```python
from build123d import *

# Parameters (mm, degrees)
BOSS_EXTRUDE1_DEPTH = 6.35
CUT_EXTRUDE2_START  = -7.35
CUT_EXTRUDE2_DEPTH  = 8.35
CIRPATTERN2_COUNT   = 8
CIRPATTERN2_ANGLE   = 180


with BuildPart() as part:
    # Sketch1 → Boss-Extrude1 (new body)
    with BuildSketch(Plane(origin=(0, 0, 0), x_dir=(0, 0, -1), z_dir=(1, 0, 0))):
        with BuildLine():
            Line((-60.325, -98.425), (-60.325, 1.27))
            ThreePointArc((-60.325, 1.27), (-12.969041148, 54.83761073), (46.001592655, 14.408164693))
            Line((46.001592655, 14.408164693), (54.245104063, -18.439722464))
            ThreePointArc((54.245104063, -18.439722464), (49.680727349, -26.131903505), (41.952464165, -21.628889834))
            Line((41.952464165, -21.628889834), (33.734959483, 9.03925515))
            ThreePointArc((33.734959483, 9.03925515), (-4.558627263, 34.626211783), (-34.925, 0))
            Line((-34.925, 0), (-34.925, -98.425))
            ThreePointArc((-34.925, -98.425), (-47.625, -111.125), (-60.325, -98.425))
        make_face()
    extrude(amount=BOSS_EXTRUDE1_DEPTH)

    # Sketch5 → Cut-Extrude2 (cut)
    with BuildSketch(Plane(origin=(6.35, 0, 0), x_dir=(0, 0, -1), z_dir=(1, 0, 0)).offset(CUT_EXTRUDE2_START)):
        Polygon((-38.1, 6.35), (-41.275, 6.35), (-41.275, 0), (-35.06174314, 0), (-35.06174314, 6.35), align=None)
    cut_extrude2 = extrude(amount=CUT_EXTRUDE2_DEPTH, mode=Mode.SUBTRACT)

    # CirPattern2: Cut-Extrude2 ×8 about axis, 4 skipped
    cirpattern2_axis = Axis((0, 0, 0), (-1, 0, 0))
    add([cut_extrude2.rotate(cirpattern2_axis, i * CIRPATTERN2_ANGLE / (CIRPATTERN2_COUNT - 1)) for i in range(1, CIRPATTERN2_COUNT) if i not in (2, 3, 4, 7)], mode=Mode.SUBTRACT)


solid = part.part
```
The listing builds one solid part. Answer for the finished solid, in the listing's coordinates (mm). A direction names the side the tool comes from. Round coordinates to 2 decimals unless told otherwise and drop trailing zeros. Write each loop counter-clockwise with the first axis right and the second up, starting at its lowest first coordinate (ties: lowest second). Pieces come first, ordered by that corner, then holes. Notation, with made-up numbers: (41.5, 38.5) -> (55.5, 38.5) arc R30 cw to (55.5, 73.5) -> close; hole circle Ø11 at (17.25, 48). An arc over 180 degrees is marked (long way). Answer as a JSON object with one key per item and string values. Group by question number.
Q1. Each of these flat-tipped pins is pushed along its axis until it touches: pin 1 Ø8 at (y, z) = (-92.5, 28) entering from -X; pin 2 Ø3 at (x, y) = (2.5, 3) entering from -Z. Where does it stop, or does it pass through?
Q2. Section C-C (y = -57) is taken. Write down the section's boundary in (x, z) (3 decimals), plus the area to 3 significant figures.
Q3. Which of the six approach directions +Z, -Z, +X, -X, +Y, -Y give full straight-line access (tool end or side, diameter ignored) to faces 4 (the face through (6.35, -15, 37)), 5 (the face through (3.131, 15.008, -38.584))?
Q4. Determine the mould class of faces 1 (the face through (3, -49, 60.325)), 2 (the face through (0, -15, 37)), 3 (the face through (3.13, 16.58, 34.43)) for opening direction Z: pulls with the +Z half, pulls with the -Z half, needs draft (parallel to the pull), parting line crosses it, or undercut.
Q5. Straight lines are drawn through the part: line 1 along Z through (x, y) = (1.25, -52) (3 decimals); line 2 along Z through (x, y) = (3.25, 14.5); line 3 along Y through (x, z) = (6.25, 29.5). For each, find the intervals that lie inside material, in ascending order.
Q6. Section A-A (x = 4) is taken. Count the separate pieces of the cut face and the enclosed holes in it, plus the area to 3 significant figures.
Q7. Section B-B (z = -5) is taken. Write down the section's boundary in (x, y), plus the area to 3 significant figures.
Check values:
{
 "1": {"pin 1": "through", "pin 2": "z = -49.24"},
 "2": {"outline": "(0, 34.925) -> (6.35, 34.925) -> (6.35, 60.325) -> (0, 60.325) -> close", "area": "161 mm^2"},
 "3": {"face 4": "+Z, -Z, +X, +Y, -Y", "face 5": "+X, -X"},
 "4": {"face 1": "pulls with the +Z half", "face 2": "needs draft", "face 3": "undercut"},
 "5": {"line 1": "34.925 to 60.325", "line 2": "-45.98 to -38.83, -31.93 to -31.77, 31.77 to 58.68", "line 3": "18.7 to 19.55, 21.25 to 50.03"},
 "6": {"separate pieces": "1", "enclosed holes": "4", "area": "5,730 mm^2"},
 "7": {"outline": "(0, 34.57) -> (6.35, 34.57) -> (6.35, 54.04) -> (0, 54.04) -> close", "area": "124 mm^2"}
}
